from build123d import *

# Parameters (mm, degrees)
EXTRUDE_1_DEPTH     = 1300
SKETCH_3_R          = 2
CUT_EXTRUDE_1_DEPTH = 1301.046633779


with BuildPart() as part:
    # 草图2 → 凸台-拉伸1 (new body)
    with BuildSketch(Plane.XY):
        with BuildLine():
            Line((-0.5, 8.5), (0.5, 8.5))
            ThreePointArc((0.5, 8.5), (2.621320344, 7.621320344), (3.5, 5.5))
            Line((3.5, 5.5), (3.5, -5.5))
            ThreePointArc((3.5, -5.5), (2.621320344, -7.621320344), (0.5, -8.5))
            Line((0.5, -8.5), (-0.5, -8.5))
            ThreePointArc((-0.5, -8.5), (-2.621320344, -7.621320344), (-3.5, -5.5))
            Line((-3.5, -5.5), (-3.5, 5.5))
            ThreePointArc((-3.5, 5.5), (-2.621320344, 7.621320344), (-0.5, 8.5))
        make_face()
    extrude(amount=EXTRUDE_1_DEPTH)

    # 草图3 → 切除-拉伸1 (cut, through all)
    with BuildSketch(Plane.ZY.offset(3.5)):
        with Locations((100, 0)):
            Circle(SKETCH_3_R)
        with Locations((200, 0)):
            Circle(SKETCH_3_R)
        with Locations((300, 0)):
            Circle(SKETCH_3_R)
        with Locations((400, 0)):
            Circle(SKETCH_3_R)
        with Locations((500, 0)):
            Circle(SKETCH_3_R)
        with Locations((600, 0)):
            Circle(SKETCH_3_R)
        with Locations((700, 0)):
            Circle(SKETCH_3_R)
        with Locations((800, 0)):
            Circle(SKETCH_3_R)
        with Locations((900, 0)):
            Circle(SKETCH_3_R)
        with Locations((1000, 0)):
            Circle(SKETCH_3_R)
    extrude(amount=-CUT_EXTRUDE_1_DEPTH, mode=Mode.SUBTRACT)


solid = part.part
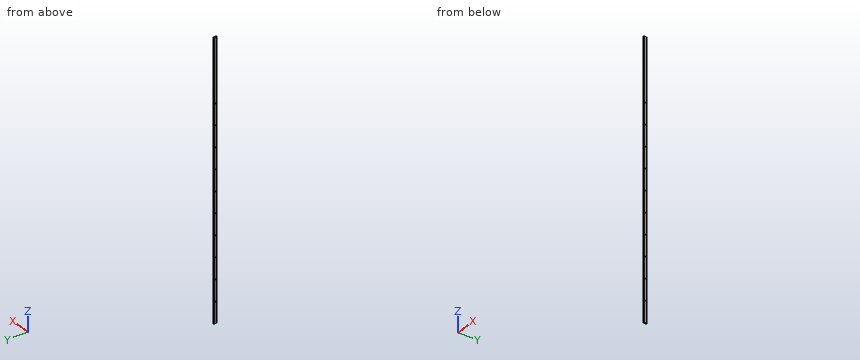
Could you check a few things on this model? Use its own coordinates, in mm. Round coordinates to 2 decimals unless told otherwise and drop trailing zeros. Loops run counter-clockwise (first coordinate to the right, second up) from the corner with the lowest first, then second, coordinate; pieces in that order, holes last. Notation, with made-up numbers: (69.25, 63.25) - (78.25, 63.25) arc R28 cw to (78.25, 95.25) - close; hole circle Ø11 at (-14.5, 36.5). An arc over 180 degrees is marked (long way). Write item = value, one per line.
1) Imagine slicing it at B-B (x = 1.75). Give the number of separate pieces and of enclosed holes in the cut face, and give its area (3 significant figures).
Computed:
separate_pieces = 1
enclosed_holes = 10
area = 21,300 mm2
2) I need wall thicknesses on line 1 along Y through (x, z) = (1.25, 700); line 2 along Y through (x, z) = (-0.75, 800); line 3 along Y through (x, z) = (-1.25, 1150). Which ranges of each line are inside material? Lowest first, please. Write a range as from..to.
Computed:
line_1 = -8.4..-2, 2..8.4
line_2 = -8.49..-2, 2..8.49
line_3 = -8.4..8.4
3) Imagine slicing it at A-A (z = 173). Please give me the cut outline in (x, y).
Computed:
outline = (-3.5, -5.5) arc R3 ccw to (-0.5, -8.5) - (0.5, -8.5) arc R3 ccw to (3.5, -5.5) - (3.5, 5.5) arc R3 ccw to (0.5, 8.5) - (-0.5, 8.5) arc R3 ccw to (-3.5, 5.5) - close
4) I'm going to push flat-ended pins straight in: P1, Ø5, axis at y = 0, z = 200, coming from the +X side; P2, Ø1.5, axis at x = -2.5, z = 1002, coming from the +Y side. Where does each tip first touch, or does it pass through?
Computed:
P1 = 3.5
P2 = 8.23
